```python
from build123d import *

# Parameters (mm, degrees)
F1_DEPTH = 0.4
F3_DEPTH = 15
F4_R     = 1.99999
F5_R     = 10


# Not quite as in the source:
# - a fillet or chamfer is up to 0.001 mm smaller than in the source, because OpenCascade refuses the exact size


with BuildPart() as f1:
    # F0 (on Top) → F1 (new body)
    with BuildSketch(Plane.XY):
        Polygon((-13, -59), (0, -59), (0, 0), (47, 0), (47, 26), (-13, 26), (-13, 0), align=None)
    extrude(amount=F1_DEPTH)

    # F2 (on face) → F3 (join)
    with BuildSketch(Plane(origin=(0, 0, 0), x_dir=(1, 0, 0), z_dir=(0, 0, -1))):
        Polygon((-13, 59), (-13, -26), (-11, -26), (47, -26), (47, -24), (-11, -24), (-11, 59), align=None)
    extrude(amount=F3_DEPTH)

    # F4 (radius 2 in the source; OpenCascade refuses exactly that, so slightly less here)
    f4_edges = [f1.edges().sort_by_distance(p)[0] for p in [
        (-11, -17.5, -15),
        (18, 24, -15),
    ]]
    fillet(f4_edges, radius=F4_R)

    # F5
    f5_edges = [f1.edges().sort_by_distance(p)[0] for p in [
        (0, -59, 0.2),
        (47, 0, 0.2),
    ]]
    fillet(f5_edges, radius=F5_R)


solid = f1.part
```
CAD build for the part. Positions are in the model's coordinates, mm. A direction names the side the tool comes from. Coordinates: 2 decimals unless noted, no trailing zeros. Order: outer loops, then holes, each group sorted by start corner. A loop starts at its lowest first (then second) coordinate and runs counter-clockwise, first axis right, second up. Notation, with made-up numbers: (-26.5, -20) - (31.5, -20) arc R13 ccw to (31.5, -10) - close; hole circle Ø3 at (80.25, 3.25). An arc over 180 degrees is marked (long way). Answer in a Markdown table with one row per item.
1. 3-axis set-ups, long thin cutter, end or side, ignore diameter. For faces 1 (the face through (16.58, 24.57, -14.4)), 2 (the face through (-12, -59, -7)): which of +Z, -Z, +X, -X, +Y, -Y reach the whole face in a straight line?
Answer:
| item | result |
|---|---|
| face 1 | -Z, +X, -Y |
| face 2 | +Z, -Z, +X, -X, -Y |
2. Slice it at C-C, the plane z = -6. List the corners of the cut face in (x, y).
Answer:
| item | result |
|---|---|
| outline | (-13, -59) - (-11, -59) - (-11, 24) - (47, 24) - (47, 26) - (-13, 26) - close |
3. Drill centre lines: L1, parallel to Y at x = -8, z = -9.75; L2, parallel to Z at x = -2.5, y = 17.5; L3, parallel to X at y = 19.5, z = -5.75. Where is each one in solid material? Low to high. Write a range as from..to.
Answer:
| item | result |
|---|---|
| L1 | 24..26 |
| L2 | 0..0.4 |
| L3 | -13..-11 |
4. Flat gauge pins, fed straight in: P1, Ø6.5, axis at y = -5, z = -8.5, coming from the +X side; P2, Ø6, axis at x = 4.5, z = -6, coming from the -Y side; P3, Ø17.5, axis at x = 13.5, y = -34, coming from the -Z side. Where does each tip first touch, or does it go through?
Answer:
| item | result |
|---|---|
| P1 | x = -11 |
| P2 | y = 24 |
| P3 | through |
